The listing builds one solid part. Answer for the finished solid, in the listing's coordinates (mm). Coordinates: 2 decimals unless noted, no trailing zeros. Write each loop counter-clockwise with the first axis right and the second up, starting at its lowest first coordinate (ties: lowest second). Pieces come first, ordered by that corner, then holes.
(1) Given P1, Ø4.5, axis at x = 210, y = 10, coming from the +Z side, flat-ended and moving along its own axis, determine where the tip first touches the part or whether it passes through.
(2) The part is cut by section C-C on x = 314.5. Determine the outline of the cut face in (y, z), plus the area to 3 significant figures.
(3) The part is cut by section B-B on y = 181. Determine the outline of the cut face in (x, z), plus the area to 4 significant figures.
(4) Straight lines are drawn through the part: line 1 (Y direction, x = 10, z = 1.35); line 2 (X direction, y = 290, z = 0.95); line 3 (X direction, y = 150, z = 0.9). For each, find the intervals that lie inside material, in ascending order.
(5) The part is cut by section A-A on z = 0.85. Determine the outline of the cut face in (x, y).
Autodesk Inventor part; units mm, degrees
ref_plane "YZ Plane" through (0, 0, 0) normal (1, 0, 0) x (0, 1, 0)
ref_plane "XZ Plane" through (0, 0, 0) normal (0, 1, 0) x (-1, 0, 0)
ref_plane "XY Plane" through (0, 0, 0) normal (0, 0, 1) x (1, 0, 0)
sketch "スケッチ1" plane through (0, 0, 0) normal (0, 0, 1) x (1, 0, 0)
  line L0 (0, 0) -> (450, 0)
  line L1 (450, 0) -> (450, 20)
  line L2 (450, 20) -> (300, 300)
  line L3 (300, 300) -> (0, 300)
  line L4 (0, 300) -> (0, 0)
  line L5 (10, 290) -> (294.0126, 290) construction
  line L6 (294.0126, 290) -> (444.0126, 10) construction
  line L7 (444.0126, 10) -> (10, 10) construction
  line L8 (10, 10) -> (10, 290) construction
  circle A0 centre (10, 290) radius 2.5
  circle A1 centre (10, 10) radius 2.5
  circle A2 centre (10, 150) radius 2.5
  circle A3 centre (210, 10) radius 2.5
  circle A4 centre (440, 10) radius 2.5
  circle A5 centre (230, 290) radius 2.5
  dimension "d0" = 300
  dimension "d1" = 450
  dimension "d2" = 300
  dimension "d3" = 20
  dimension "d6" = 10
  dimension "d7" = 5
  dimension "d8" = 10
  dimension "d9" = 200
  dimension "d10" = 220
extrude "押し出し1" add sketch "スケッチ1" along normal blind 2
fillet "フィレット1" radius 5 5 edges at (450, 0, 1) (450, 20, 1) (0, 0, 1) (300, 300, 1) (0, 300, 1)
properties part number "防水1" material "PET プラスチック"
Model answer:
1. P1: passes through
2. outline: (0, 0) - (272.93, 0) - (272.93, 2) - (0, 2) - close
2. area: 546 mm2
3. outline: (0, 0) - (363.75, 0) - (363.75, 2) - (0, 2) - close
3. area: 727.5 mm2
4. line 1: y = 0 to 7.5, 12.5 to 147.5, 152.5 to 287.5, 292.5 to 300
4. line 2: x = 0 to 7.5, 12.5 to 227.5, 232.5 to 305.36
4. line 3: x = 0 to 7.5, 12.5 to 380.36
5. outline: (0, 5) arc R5 ccw to (5, 0) - (445, 0) arc R5 ccw to (450, 5) - (450, 18.75) arc R5 ccw to (449.41, 21.11) - (301.41, 297.36) arc R5 ccw to (297.01, 300) - (5, 300) arc R5 ccw to (0, 295) - close; hole circle Ø5 at (10, 10); hole circle Ø5 at (10, 150); hole circle Ø5 at (10, 290); hole circle Ø5 at (210, 10); hole circle Ø5 at (230, 290); hole circle Ø5 at (440, 10)
